The model under review builds one solid part; all positions refer to its coordinate system, in mm. Face numbers are marked on the shaded views. A direction names the side the tool comes from. Coordinates: 2 decimals unless noted, no trailing zeros. Loops run counter-clockwise (first coordinate to the right, second up) from the corner with the lowest first, then second, coordinate; pieces in that order, holes last. Notation, with made-up numbers: M 12.25,72.5 L 22.25,72.5 A13 ccw 22.25,92.5 Z; hole C 17,17 d6. An arc over 180 degrees is marked long. Return JSON: item names as keys, results as strings.
```python
from build123d import *

# Parameters (mm, degrees)
HOLE_WIZARD_M10_1_D           = 8.5
HOLE_WIZARD_M10_1_DEPTH       = 12
HOLE_WIZARD_M10_1_CSINK_D     = 10.05
HOLE_WIZARD_M10_1_CSINK_ANGLE = 90
HOLE_WIZARD_M10_1_TIP         = 2.553657631
CHAMFER_1_SIZE                = 3
HOLE_WIZARD_M3_1_D            = 2.5
HOLE_WIZARD_M3_1_DEPTH        = 7.5
HOLE_WIZARD_M3_1_CSINK_D      = 3.05
HOLE_WIZARD_M3_1_CSINK_ANGLE  = 90
HOLE_WIZARD_M3_1_TIP          = 0.751075774
CHAMFER_2_SIZE                = 0.5


with BuildPart() as part:
    # 草图1 → 旋转1 (revolve)
    with BuildSketch(Plane(origin=(0, 0, 0), x_dir=(0, 0, -1), z_dir=(1, 0, 0)), mode=Mode.PRIVATE) as revolve_1_sk:
        Polygon((0, 0), (0, 25), (5, 25), (5, 12.5), (20, 12.5), (20, 0), align=None)
    revolve(revolve_1_sk.sketch.rotate(Axis((0, 0, 109.85915493), (0, 0, -1)), 90), axis=Axis((0, 0, 109.85915493), (0, 0, -1)))

    # M10 螺纹孔1
    with Locations(Plane(origin=(0, 0, -20), x_dir=(-1, 0, 0), z_dir=(0, 0, -1))):
        with Locations((0, 0)):
            CounterSinkHole(HOLE_WIZARD_M10_1_D / 2, HOLE_WIZARD_M10_1_CSINK_D / 2, depth=HOLE_WIZARD_M10_1_DEPTH, counter_sink_angle=HOLE_WIZARD_M10_1_CSINK_ANGLE)
            with Locations((0, 0, -(HOLE_WIZARD_M10_1_DEPTH + HOLE_WIZARD_M10_1_TIP / 2))):  # 118° drill point
                Cone(0, HOLE_WIZARD_M10_1_D / 2, HOLE_WIZARD_M10_1_TIP, mode=Mode.SUBTRACT)

    # 倒角1
    chamfer_1_edges = [part.edges().sort_by_distance(p)[0] for p in [
        (-12.5, 0, -5),
    ]]
    chamfer(chamfer_1_edges, length=CHAMFER_1_SIZE)

    # M3 螺纹孔1
    with Locations(Plane.XY):
        with Locations((-20, 0), (0, 20), (20, 0), (0, -20)):
            CounterSinkHole(HOLE_WIZARD_M3_1_D / 2, HOLE_WIZARD_M3_1_CSINK_D / 2, depth=HOLE_WIZARD_M3_1_DEPTH, counter_sink_angle=HOLE_WIZARD_M3_1_CSINK_ANGLE)
            with Locations((0, 0, -(HOLE_WIZARD_M3_1_DEPTH + HOLE_WIZARD_M3_1_TIP / 2))):  # 118° drill point
                Cone(0, HOLE_WIZARD_M3_1_D / 2, HOLE_WIZARD_M3_1_TIP, mode=Mode.SUBTRACT)

    # 倒角2
    chamfer_2_edges = [part.edges().sort_by_distance(p)[0] for p in [
        (-12.5, 0, -20),
        (-25, 0, 0),
    ]]
    chamfer(chamfer_2_edges, length=CHAMFER_2_SIZE)


solid = part.part
```
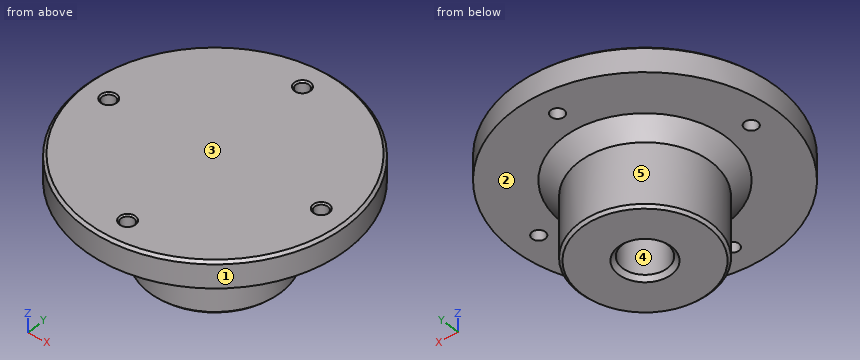
1. Add section B-B on z = -12.5. Give the boundary of the cut face in (x, y), plus the area to 3 significant figures.
Check values:
{"outline": "C 0,0 d25; hole C 0,0 d8.5", "area": "434 mm²"}
2. Add section C-C on z = -7. Give the boundary of the cut face in (x, y), plus the area to 3 significant figures.
Check values:
{"outline": "C 0,0 d27; hole C 0,0 d5.17", "area": "552 mm²"}
3. Add section A-A on z = -3. Give the boundary of the cut face in (x, y).
Check values:
{"outline": "C 0,0 d50; hole C -20,0 d2.5; hole C 0,-20 d2.5; hole C 0,20 d2.5; hole C 20,0 d2.5"}
4. The part is to be moulded in two halves that separate along X. For the marked faces 3, 4 and 5, say which applies: released by +X, released by -X, zero draft, split by the parting line, or undercut.
Check values:
{"face 3": "zero draft", "face 4": "undercut", "face 5": "split by the parting line"}
5. Machinability: for the marked faces 1 and 2, which of the approach directions +Z, -Z, +X, -X, +Y, -Y give a long, thin tool a straight path to every point of the face, cutting with its end or side? Answer none if there is none.
Check values:
{"face 1": "+Z, -Z", "face 2": "-Z"}
6. To check wall thickness, follow line 1 (Y direction, x = 0, z = -2.3); line 2 (X direction, y = 1, z = -3.5); line 3 (Z direction, x = -21, y = -4). State the ranges of each line that lie inside material, in increasing order.
Check values:
{"line 1": "-25 to -21.25, -18.75 to 18.75, 21.25 to 25", "line 2": "-24.98 to -20.75, -19.25 to 19.25, 20.75 to 24.98", "line 3": "-5 to 0"}
7. Insertion check: pin 1 Ø2 at (x, y) = (-4, 17) entering from -Z; pin 2 Ø1.5 at (y, z) = (12, -11.5) entering from +X; pin 3 Ø3 at (x, y) = (9.5, 11) entering from -Z. Each pin has a flat end and moves straight along its axis. Give the tip position at first contact, or say it passes through.
Check values:
{"pin 1": "z = -5", "pin 2": "x = 5.45", "pin 3": "z = -7.47"}
